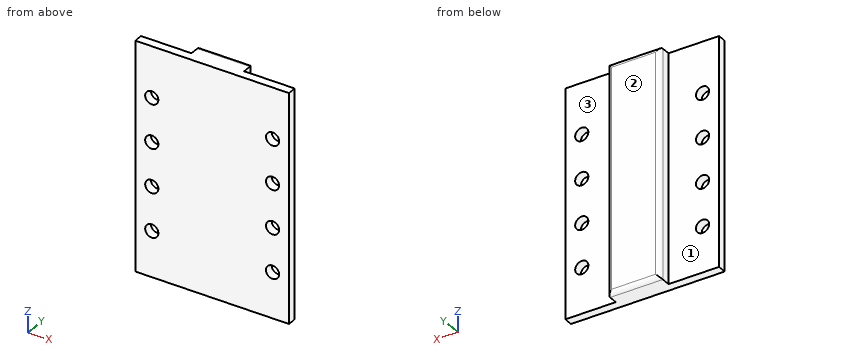
from build123d import *

# Parameters (mm, degrees)
SKETCH_1_W                  = 35
SKETCH_1_H                  = 52
EXTRUDE_1_DEPTH             = 2
EXTRUDE_2_REACH             = 33.405
SKETCH_2_W                  = 12
SKETCH_2_H                  = 3
EXTRUDE_2_DIRECTION_2_REACH = 33.405
SKETCH_3_R                  = 1.5
CUT_EXTRUDE_1_DEPTH         = 10
FILLET_1_R                  = 1


with BuildPart() as part:
    # Эскиз1 → Бобышка-Вытянуть1 (new body)
    with BuildSketch(Plane(origin=(0, 0, 0), x_dir=(1, 0, 0), z_dir=(0, 1, 0))):
        Rectangle(SKETCH_1_W, SKETCH_1_H)
    extrude(amount=EXTRUDE_1_DEPTH)

    # Бобышка-Вытянуть2: up to this face of the body (flat: up to its plane)
    extrude_2_end = Plane(part.part.faces().sort_by_distance((0, 1, 26))[0])
    # Эскиз2 → Бобышка-Вытянуть2 (add, up to the picked face)
    with BuildSketch(Plane.XY, mode=Mode.PRIVATE) as extrude_2_sk1:
        with Locations((0, 3.5)):
            Rectangle(SKETCH_2_W, SKETCH_2_H)
    extrude_2_tool1 = split(extrude(extrude_2_sk1.sketch, amount=EXTRUDE_2_REACH, mode=Mode.PRIVATE), bisect_by=extrude_2_end, keep=Keep.BOTH, mode=Mode.PRIVATE)
    add(extrude_2_tool1.solids().sort_by(Axis((0, 3.5, 0), (0, 0, 1)))[0])

    # Бобышка-Вытянуть2 direction 2: up to this face of the body (flat: up to its plane)
    extrude_2_direction_2_end = Plane(part.part.faces().sort_by_distance((0, 1, -26))[0])
    # Эскиз2 → Бобышка-Вытянуть2 direction 2 (add, up to the picked face)
    with BuildSketch(Plane.XY, mode=Mode.PRIVATE) as extrude_2_direction_2_sk1:
        with Locations((0, 3.5)):
            Rectangle(SKETCH_2_W, SKETCH_2_H)
    extrude_2_direction_2_tool1 = split(extrude(extrude_2_direction_2_sk1.sketch, amount=-EXTRUDE_2_DIRECTION_2_REACH, mode=Mode.PRIVATE), bisect_by=extrude_2_direction_2_end, keep=Keep.BOTH, mode=Mode.PRIVATE)
    add(extrude_2_direction_2_tool1.solids().sort_by(Axis((0, 3.5, 0), (0, 0, -1)))[0])

    # Эскиз3 → Вырез-Вытянуть1 (cut)
    with BuildSketch(Plane(origin=(0, 2, 0), x_dir=(1, 0, 0), z_dir=(0, 1, 0))):
        with Locations(Location((13.75, 15.6, 0), (0, 0, 270))):
            Circle(SKETCH_3_R)
        with Locations(Location((-13.75, 15.6, 0), (0, 0, 270))):
            Circle(SKETCH_3_R)
        with Locations(Location((-13.75, 5.6, 0), (0, 0, 270))):
            Circle(SKETCH_3_R)
        with Locations(Location((13.75, 5.6, 0), (0, 0, 270))):
            Circle(SKETCH_3_R)
        with Locations(Location((-13.75, -4.4, 0), (0, 0, 270))):
            Circle(SKETCH_3_R)
        with Locations(Location((13.75, -4.4, 0), (0, 0, 270))):
            Circle(SKETCH_3_R)
        with Locations(Location((-13.75, -14.4, 0), (0, 0, 270))):
            Circle(SKETCH_3_R)
        with Locations(Location((13.75, -14.4, 0), (0, 0, 270))):
            Circle(SKETCH_3_R)
    extrude(amount=-CUT_EXTRUDE_1_DEPTH, mode=Mode.SUBTRACT)

    # Скругление1
    fillet_1_edges = [part.edges().sort_by_distance(p)[0] for p in [
        (0, 5, 26),
        (6, 5, 0),
        (-6, 5, 0),
        (0, 5, -26),
    ]]
    fillet(fillet_1_edges, radius=FILLET_1_R)


solid = part.part
Work out the finished part from the listing and answer in its coordinate system (mm). Face numbers are marked on the shaded views. A direction names the side the tool comes from. Give positions to 0.01 mm unless a question says otherwise; leave off trailing zeros. Loops run counter-clockwise (first coordinate to the right, second up) from the corner with the lowest first, then second, coordinate; pieces in that order, holes last. Notation, with made-up numbers: (1, 53) - (24, 53) arc R16 ccw to (24, 64) - close; hole circle Ø2 at (-33.75, 72.25). An arc over 180 degrees is marked (long way). Answer in a Markdown table with one row per item. Add a question column.
Q1. The part is cut by section C-C (y = 1). State how many separate pieces and enclosed holes the cut face has, and give its area (3 significant figures).
Q2. The part is cut by section B-B (x = -13.75). Determine the outline of the cut face in (y, z), and give its area (3 significant figures).
Q3. A tool of negligible diameter and unlimited length cuts with its end or side. For the marked faces 1, 2 and 3, from which of +Z, -Z, +X, -X, +Y, -Y can it reach the whole face along a straight path? Write none if from no direction.
Q4. The part is cut by section D-D (z = -2). Determine the outline of the cut face in (x, y).
Q5. Each of these flat-tipped pins is pushed along its axis until it touches: P1, Ø1.5, axis at x = 12.5, z = 0, coming from the -Y side; P2, Ø3.5, axis at x = 10.5, z = -12, coming from the +Y side; P3, Ø2.5, axis at x = 13.75, z = -5.6, coming from the -Y side. Where does it stop, or does it pass through?
Q6. Consider line 1 along X through (y, z) = (0.65, -15.6); line 2 along Y through (x, z) = (-11, 22); line 3 along X through (y, z) = (2.9, -15). Determine where each line is inside the solid, lowest interval first.
Q7. The part is cut by section A-A (z = 4.4). Determine the outline of the cut face in (x, y), and give its area (3 significant figures).
Solution:
| question | item | result |
|---|---|---|
| 1 | separate pieces | 1 |
| 1 | enclosed holes | 8 |
| 1 | area | 1,760 mm² |
| 2 | outline | (0, -26) - (2, -26) - (2, -17.1) - (0, -17.1) - close; (0, -14.1) - (2, -14.1) - (2, -7.1) - (0, -7.1) - close; (0, -4.1) - (2, -4.1) - (2, 2.9) - (0, 2.9) - close; (0, 5.9) - (2, 5.9) - (2, 12.9) - (0, 12.9) - close; (0, 15.9) - (2, 15.9) - (2, 26) - (0, 26) - close |
| 2 | area | 80.0 mm² |
| 3 | face 1 | +Z, -Z, -X, +Y |
| 3 | face 2 | +Z, -Z, +X, -X, +Y |
| 3 | face 3 | +Z, -Z, +X, +Y |
| 4 | outline | (-17.5, 0) - (17.5, 0) - (17.5, 2) - (6, 2) - (6, 4) arc R1 ccw to (5, 5) - (-5, 5) arc R1 ccw to (-6, 4) - (-6, 2) - (-17.5, 2) - close |
| 5 | P1 | stops at y = 0 |
| 5 | P2 | stops at y = 2 |
| 5 | P3 | passes through |
| 6 | line 1 | x = -17.5 to -15.25, -12.25 to 12.25, 15.25 to 17.5 |
| 6 | line 2 | y = 0 to 2 |
| 6 | line 3 | x = -6 to 6 |
| 7 | outline | (-17.5, 0) - (-15.25, 0) - (-15.25, 2) - (-17.5, 2) - close; (-12.25, 0) - (12.25, 0) - (12.25, 2) - (6, 2) - (6, 4) arc R1 ccw to (5, 5) - (-5, 5) arc R1 ccw to (-6, 4) - (-6, 2) - (-12.25, 2) - close; (15.25, 0) - (17.5, 0) - (17.5, 2) - (15.25, 2) - close |
| 7 | area | 93.6 mm² |
